Input: part model. Units: mm. Frame: model coordinates. Face numbers are marked on the shaded views. A direction names the side the tool comes from. Round coordinates to 2 decimals unless told otherwise and drop trailing zeros. Loops run counter-clockwise (first coordinate to the right, second up) from the corner with the lowest first, then second, coordinate; pieces in that order, holes last.
(1) Cut plane B-B, the plane z = -10. Output: boundary loops of the cut face in (x, y).
(2) Cut plane C-C, the plane y = 0. Output: boundary loops of the cut face in (x, z), and give its area (3 significant figures).
(3) Cut plane A-A, the plane y = -15.75. Output: boundary loops of the cut face in (x, z), and give its area (3 significant figures).
(4) Line query: line 1 (Y direction, x = 0.6, z = -10); line 2 (Y direction, x = 2.3, z = -1.5); line 3 (Y direction, x = 1, z = -6.75). Output: solid intervals per line, ascending.
(5) Access query for the marked faces 1, 2, 3 and 4. Directions: +Z, -Z, +X, -X, +Y, -Y. A direction counts if a zero-diameter tool reaches every point of the face in a straight line with its end or side. Return the directions, or none.
(6) Cut plane D-D, the plane x = 1.75. Output: boundary loops of the cut face in (y, z), and give its area (3 significant figures).
(7) First-contact query: pin 1 Ø8.5 at (y, z) = (0, 0) entering from +X; pin 2 Ø0.6 at (x, z) = (1, -9.5) entering from -Y; pin 3 Ø7.5 at (y, z) = (-64, -1.5) entering from -X. Flat tips, straight axial feed; report the tip coordinate or a pass-through.
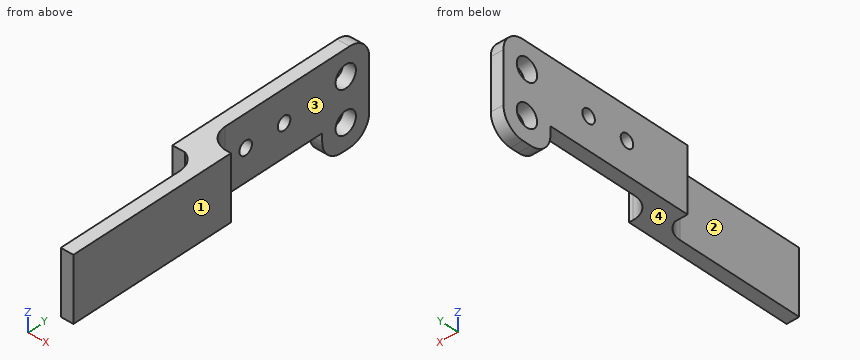
from build123d import *

# Parameters (mm, degrees)
SKETCH1_W           = 22
SKETCH1_H           = 12
SKETCH1_R           = 2.6
BOSS_EXTRUDE1_DEPTH = 3
SKETCH2_W           = 15
SKETCH2_H           = 36
BOSS_EXTRUDE2_DEPTH = 3
FILLET1_R           = 5
FILLET2_R           = 1
SKETCH4_W           = 15
SKETCH4_H           = 34.286255804
BOSS_EXTRUDE3_DEPTH = 12.2
SKETCH7_W           = 12.2
SKETCH7_H           = 15
CUT_EXTRUDE3_DEPTH  = 50
SKETCH8_R           = 1.6
CUT_EXTRUDE4_DEPTH  = 10
SKETCH9_W           = 15
SKETCH9_H           = 5.23
BOSS_EXTRUDE4_DEPTH = 6
SKETCH10_W          = 3
SKETCH10_H          = 15
BOSS_EXTRUDE5_DEPTH = 35
FILLET3_R           = 5
FILLET4_R           = 5
SKETCH11_W          = 15.033805152
SKETCH11_H          = 2.020668066
CUT_EXTRUDE5_DEPTH  = 3


with BuildPart() as part:
    # Sketch1 → Boss-Extrude1 (new body)
    with BuildSketch(Plane(origin=(0, 0, 0), x_dir=(0, 0, -1), z_dir=(1, 0, 0))):
        with Locations((5, 0)):
            Rectangle(SKETCH1_W, SKETCH1_H)
        with Locations((10, 0)):
            Circle(SKETCH1_R, mode=Mode.SUBTRACT)
        Circle(SKETCH1_R, mode=Mode.SUBTRACT)
    extrude(amount=BOSS_EXTRUDE1_DEPTH)

    # Sketch2 → Boss-Extrude2 (add)
    with BuildSketch(Plane(origin=(0, 0, 0), x_dir=(0, 0, -1), z_dir=(1, 0, 0))):
        with Locations((1.5, -24)):
            Rectangle(SKETCH2_W, SKETCH2_H)
    extrude(amount=BOSS_EXTRUDE2_DEPTH)

    # Fillet1
    fillet1_edges = [part.edges().sort_by_distance(p)[0] for p in [
        (1.5, -6, -16),
        (1.5, 6, 6),
        (1.5, 6, -16),
    ]]
    fillet(fillet1_edges, radius=FILLET1_R)

    # Fillet2
    fillet2_edges = [part.edges().sort_by_distance(p)[0] for p in [
        (1.5, -42, 6),
        (1.5, -42, -9),
    ]]
    fillet(fillet2_edges, radius=FILLET2_R)

    # Sketch4 → Boss-Extrude3 (add)
    with BuildSketch(Plane(origin=(3, 0, 0), x_dir=(0, 0, -1), z_dir=(1, 0, 0))):
        with Locations((1.5, -23.856872098)):
            Rectangle(SKETCH4_W, SKETCH4_H)
    extrude(amount=BOSS_EXTRUDE3_DEPTH)

    # Sketch7 → Cut-Extrude3 (cut)
    with BuildSketch(Plane(origin=(0, -6.713744196, 0), x_dir=(1, 0, 0), z_dir=(0, 1, 0))):
        with Locations((9.1, 1.5)):
            Rectangle(SKETCH7_W, SKETCH7_H)
    extrude(amount=-CUT_EXTRUDE3_DEPTH, mode=Mode.SUBTRACT)

    # Sketch8 → Cut-Extrude4 (cut)
    with BuildSketch(Plane(origin=(3, 0, 0), x_dir=(0, 0, -1), z_dir=(1, 0, 0))):
        with Locations((1.5, -15.75)):
            Circle(SKETCH8_R)
        with Locations((1.5, -25.55)):
            Circle(SKETCH8_R)
    extrude(amount=-CUT_EXTRUDE4_DEPTH, mode=Mode.SUBTRACT)

    # Sketch9 → Boss-Extrude4 (add)
    with BuildSketch(Plane(origin=(3, 0, 0), x_dir=(0, 0, -1), z_dir=(1, 0, 0))):
        with Locations((1.5, -38.385)):
            Rectangle(SKETCH9_W, SKETCH9_H)
    extrude(amount=BOSS_EXTRUDE4_DEPTH)

    # Sketch10 → Boss-Extrude5 (add)
    with BuildSketch(Plane(origin=(0, -41, 0), x_dir=(-1, 0, 0), z_dir=(0, -1, 0))):
        with Locations((-7.5, 1.5)):
            Rectangle(SKETCH10_W, SKETCH10_H)
    extrude(amount=BOSS_EXTRUDE5_DEPTH)

    # Fillet3
    # the kernel refuses this fillet: 5 mm, written as the material it adds along each edge
    with BuildSketch(Plane(origin=(6, -41, 6), x_dir=(0, -1, 0), z_dir=(0, 0, -1))) as fillet3_piece_1:
        with BuildLine():
            CenterArc((4.582575695, 5), FILLET3_R, 203.578178478, 66.421821522)
            Line((0, 3), (-0.091651514, 2.96))
            ThreePointArc((-0.091651514, 2.96), (-0.1, 1.5), (-0.1, 0))
            Line((-0.1, 0), (0, -0.1))
            Line((0, -0.1), (4.582575695, -0.1))
            Line((4.582575695, -0.1), (4.582575695, 0))
        make_face()
    extrude(amount=15)

    # Fillet4
    fillet4_edges = [part.edges().sort_by_distance(p)[0] for p in [
        (3, -35.77, -1.5),
    ]]
    fillet(fillet4_edges, radius=FILLET4_R)

    # Sketch11 → Cut-Extrude5 (cut)
    with BuildSketch(Plane(origin=(3, 0, 0), x_dir=(0, 0, -1), z_dir=(1, 0, 0))):
        with Locations((1.516902576, -42.010334033)):
            Rectangle(SKETCH11_W, SKETCH11_H)
    extrude(amount=-CUT_EXTRUDE5_DEPTH, mode=Mode.SUBTRACT)


solid = part.part
Reported:
1. outline: (0, -6) - (3, -6) - (3, -2.6) - (0, -2.6) - close; (0, 2.6) - (3, 2.6) - (3, 6) - (0, 6) - close
2. outline: (0, -16) - (3, -16) - (3, -12.6) - (0, -12.6) - close; (0, -7.4) - (3, -7.4) - (3, -2.6) - (0, -2.6) - close; (0, 2.6) - (3, 2.6) - (3, 6) - (0, 6) - close
2. area: 34.8 mm2
3. outline: (0, -9) - (3, -9) - (3, -3.1) - (0, -3.1) - close; (0, 0.1) - (3, 0.1) - (3, 6) - (0, 6) - close
3. area: 35.4 mm2
4. line 1: y = -6 to -2.6, 2.6 to 6
4. line 2: y = -41 to -27.15, -23.95 to -17.35, -14.15 to -2.12, 2.12 to 6
4. line 3: y = -41 to 6
5. face 1: +Z, -Z, +X, +Y, -Y
5. face 2: +Z, -Z, -X, -Y
5. face 3: +Z, -Z, +X, +Y
5. face 4: -Z, +X, -X, -Y
6. outline: (-41, -9) - (-6, -9) - (-6, -11) arc R5 ccw to (-1, -16) - (1, -16) arc R5 ccw to (6, -11) - (6, 1) arc R5 ccw to (1, 6) - (-41, 6) - close; hole circle Ø3.2 at (-25.55, -1.5); hole circle Ø3.2 at (-15.75, -1.5); hole circle Ø5.2 at (0, -10); hole circle Ø5.2 at (0, 0)
6. area: 714 mm2
7. pin 1: stops at x = 3
7. pin 2: stops at y = -6
7. pin 3: stops at x = 6
